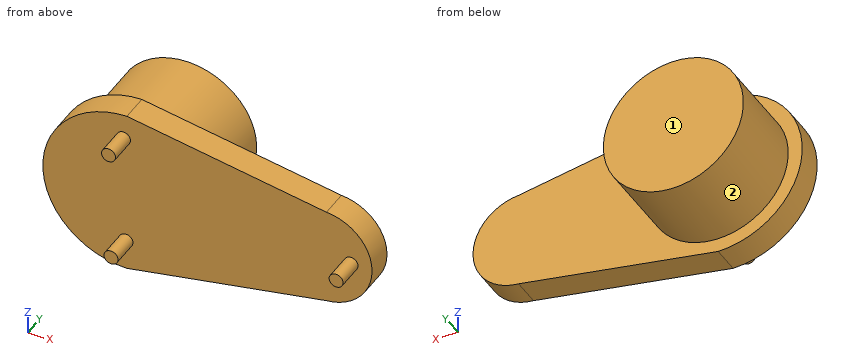
Autodesk Inventor part; units mm, degrees
ref_plane "YZ Plane" through (0, 0, 0) normal (1, 0, 0) x (0, 1, 0)
ref_plane "XZ Plane" through (0, 0, 0) normal (0, 1, 0) x (-1, 0, 0)
ref_plane "XY Plane" through (0, 0, 0) normal (0, 0, 1) x (1, 0, 0)
sketch "Skizze1" plane through (0, 0, 0) normal (0, 1, 0) x (-1, 0, 0)
  circle A0 centre (9.2308, -70.3479) radius 17.5
  arc A1 (79.2308, -100.3479) -> (79.2308, -40.3479) centre (79.2308, -70.3479) ccw
  line L0 (79.2308, -40.3479) -> (8.002, -52.8911)
  line L1 (79.2308, -100.3479) -> (7.9966, -87.8043)
  circle A2 centre (79.2308, -70.3479) radius 20
  point P0 (0, 0)
  dimension "d1" = 35
  dimension "d20" = 30
  dimension "d21" = 70
  dimension "d22" = 0
  dimension "d24" = 40
extrude "Extrusion1" add sketch "Skizze1" along normal blind 10 contours A0 | A0 L0 A1 L1 | A2
sketch "Skizze2" plane through (0, 10, 0) normal (0, 1, 0) x (1, 0, 0)
  arc A0 (-79.2308, 100.3479) -> (-79.2308, 40.3479) centre (-79.2308, 70.3479) ccw
  circle A1 centre (-79.2308, 70.3479) radius 25
  point P0 (0, 0)
  dimension "d23" = 50
extrude "Extrusion2" add sketch "Skizze2" along normal blind 30
sketch "Skizze3" plane through (0, 0, 0) normal (0, -1, 0) x (1, 0, 0)
  circle A0 centre (-79.56, -89.4817) radius 2.5
  circle A1 centre (-80.4525, -49.4817) radius 2.5
  circle A2 centre (0.7692, -70.1017) radius 2.5
  arc A3 (-8.002, -52.8911) -> (-8.002, -52.8911) centre (-9.2308, -70.3479) ccw
  point P0 (0, 0)
  point P1 (-8.4112, -91.1215)
  point P2 (-79.56, -69.4817)
  dimension "d7" = 5
  dimension "d8" = 5
  dimension "d9" = 5
  dimension "d10" = 10
  dimension "d11" = 20
  dimension "d12" = 0
  dimension "d13" = 20
extrude "Extrusion3" add sketch "Skizze3" along normal blind 10 contours A0 | A1 | A2
properties part number "LIDAR-Sensor"
For this review, take the finished solid that the model builds, in its own axes (mm). Face numbers are marked on the shaded views. A direction names the side the tool comes from. Round coordinates to 2 decimals unless told otherwise and drop trailing zeros. Write each loop counter-clockwise with the first axis right and the second up, starting at its lowest first coordinate (ties: lowest second). Pieces come first, ordered by that corner, then holes. Notation, with made-up numbers: (41, -17.5) - (92, -17.5) arc R30 ccw to (92, 17.5) - close; hole circle Ø10 at (-13, 13). An arc over 180 degrees is marked (long way). Write each question's results on one line, items separated by ' | '.
Item 1: To check wall thickness, follow line 1 along Y through (x, z) = (-21.5, -81); line 2 along X through (y, z) = (4, -71); line 3 along Y through (x, z) = (-103, -75.5). State the ranges of each line that lie inside material, in increasing order. Write a range as from..to.
Calculated:
line 1: y = 0..10 | line 2: x = -109.22..8.26 | line 3: y = 0..40
Item 2: Take a section at D-D on y = 15.5. State the section outline as (x, z) points.
Calculated:
outline: circle Ø50 at (-79.23, -70.35)
Item 3: For pin 1 (5 mm diameter, centred on y = 8.5, z = -78, fed in from +X); pin 2 (5 mm diameter, centred on x = -13, z = -72.5, fed in from -Y); pin 3 (10 mm diameter, centred on y = 4.5, z = -54.5, fed in from +X), all flat-tipped, find the tip position at first contact; note any pin that passes through.
Calculated:
pin 1: stops at x = 7.49 | pin 2: stops at y = 0 | pin 3: stops at x = 4.5
Item 4: Take a section at C-C on y = -6. State the section outline as (x, z) points.
Calculated:
outline: circle Ø5 at (-80.45, -49.48); circle Ø5 at (-79.56, -89.48); circle Ø5 at (0.77, -70.1)
Item 5: Take a section at B-B on x = -62. State the section outline as (y, z) points, then the cut area to 3 significant figures.
Calculated:
outline: (0, -97.31) - (10, -97.31) - (10, -88.46) - (40, -88.46) - (40, -52.23) - (10, -52.23) - (10, -43.38) - (0, -43.38) - close | area: 1,630 mm^2
Item 6: For the marked faces 1 and 2, list the 3-axis set-ups (+Z, -Z, +X, -X, +Y, -Y) from which the entire face can be reached by the end or side of a thin tool; tool diameter is ignored.
Calculated:
face 1: +Z, -Z, +X, -X, +Y | face 2: +Y
Item 7: Take a section at A-A on z = -78. State the section outline as (x, y) points, then the cut area to 3 significant figures.
Calculated:
outline: (-108.24, 0) - (6.51, 0) - (6.51, 10) - (-55.43, 10) - (-55.43, 40) - (-103.03, 40) - (-103.03, 10) - (-108.24, 10) - close | area: 2,580 mm^2
